Part model, mm, in its own coordinate system. Face numbers are marked on the shaded views. A direction names the side the tool comes from. Round coordinates to 2 decimals unless told otherwise and drop trailing zeros. Loops run counter-clockwise (first coordinate to the right, second up) from the corner with the lowest first, then second, coordinate; pieces in that order, holes last.
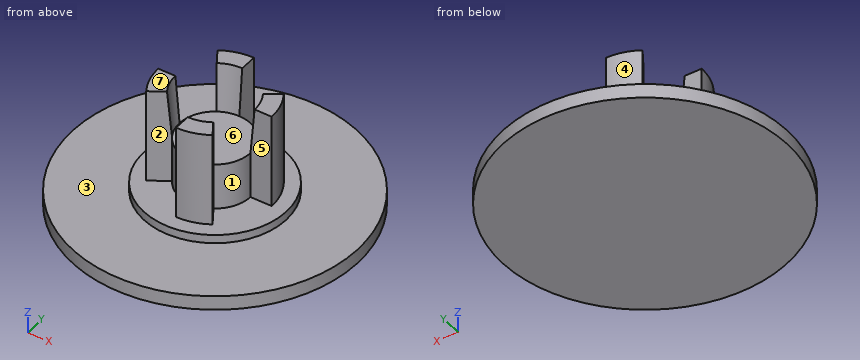
from build123d import *

# Parameters (mm, degrees)
F3_DEPTH = 6.6
F4_COUNT = 4
F5_DEPTH = 3.35
F5_TAPER = -5


with BuildPart() as f1:
    # F0 (on Front) → F1 (revolve)
    with BuildSketch(Plane.XZ):
        Polygon((0, 4.85), (0, 0), (10, 0), (10, 1), (5, 1), (5, 1.6), (2.5, 1.6), (2.5, 3.85), (2.5, 4.85), align=None)
    revolve(axis=Axis((0, 0, 2.425), (0, 0, -1)))

    # F2 (on face) → F3 (join)
    with BuildSketch(Plane.XY.offset(1.6)):
        with BuildLine():
            ThreePointArc((4, 0), (3.8409617055, 1.1166974421), (3.3764934114, 2.1445960558))
            Line((3.3764934114, 2.1445960558), (2.1103083822, 1.3403725349))
            ThreePointArc((2.1103083822, 1.3403725349), (2.4006010659, 0.6979359013), (2.5, 0))
            Line((2.5, 0), (4, 0))
        make_face()
    extrude(amount=F3_DEPTH)

    # F4: F1 ×4 about axis
    f4_axis = Axis((0, 0, 2.425), (0, 0, -1))


with BuildPart() as f1_1:
    add(f1.part)
    for i in range(1, F4_COUNT):
        add(f1.part.rotate(f4_axis, i * 360 / F4_COUNT))

    # F1_face1 (on face) → F5 (cut, through all)
    with BuildSketch(Plane.XY.offset(4.85)):
        with BuildLine():
            ThreePointArc((1.3403725349, -2.1103083822), (2.1909965013, -1.203966084), (2.5, 0))
            ThreePointArc((2.5, 0), (2.4006010659, 0.6979359013), (2.1103083822, 1.3403725349))
            ThreePointArc((2.1103083822, 1.3403725349), (1.203966084, 2.1909965013), (0, 2.5))
            ThreePointArc((0, 2.5), (-0.6979359013, 2.4006010659), (-1.3403725349, 2.1103083822))
            ThreePointArc((-1.3403725349, 2.1103083822), (-2.1909965013, 1.203966084), (-2.5, 0))
            ThreePointArc((-2.5, 0), (-2.4006010659, -0.6979359013), (-2.1103083822, -1.3403725349))
            ThreePointArc((-2.1103083822, -1.3403725349), (-1.203966084, -2.1909965013), (0, -2.5))
            ThreePointArc((0, -2.5), (0.6979359013, -2.4006010659), (1.3403725349, -2.1103083822))
        make_face()
    extrude(amount=F5_DEPTH, taper=F5_TAPER, mode=Mode.SUBTRACT)


solid = f1_1.part
1) Slice it at A-A, the plane z = 4. Give the cut face in (x, y).
Values:
outline: (-4, 0) arc R4 ccw to (-3.38, -2.14) - (-2.11, -1.34) arc R2.5 ccw to (0, -2.5) - (0, -4) arc R4 ccw to (2.14, -3.38) - (1.34, -2.11) arc R2.5 ccw to (2.5, 0) - (4, 0) arc R4 ccw to (3.38, 2.14) - (2.11, 1.34) arc R2.5 ccw to (0, 2.5) - (0, 4) arc R4 ccw to (-2.14, 3.38) - (-1.34, 2.11) arc R2.5 ccw to (-2.5, 0) - close
2) Tool access for the marked faces 5, 6 and 7: list every direction of +Z, -Z, +X, -X, +Y, -Y with a clear straight run to the whole face (end or side of a thin tool).
Values:
face 5: +Z, +X, -Y
face 6: +Z
face 7: +Z, +X, -X, +Y, -Y
3) Slice it at D-D, the plane x = -6.75. Give the cut face in (y, z), then the cut area to 3 significant figures.
Values:
outline: (-7.38, 0) - (7.38, 0) - (7.38, 1) - (-7.38, 1) - close
area: 14.8 mm2
4) Drop flat-ended pins along their axis: pin 1 Ø4 at (x, z) = (-1.5, 7) entering from -Y; pin 2 Ø1.7 at (x, z) = (-3.5, 5.5) entering from +Y; pin 3 Ø2 at (x, y) = (-3.5, 2) entering from +Z. Give the stop position or say it passes through.
Values:
pin 1: stops at y = -4
pin 2: stops at y = 0
pin 3: stops at z = 1.6
5) Slice it at C-C, the plane x = 5.25. Give the cut face in (y, z).
Values:
outline: (-8.51, 0) - (8.51, 0) - (8.51, 1) - (-8.51, 1) - close
6) Slice it at B-B, the plane z = 5.75. Give the number of separate pieces and of enclosed holes in the cut face, then the cut area to 3 significant figures.
Values:
separate pieces: 4
enclosed holes: 0
area: 10.6 mm2
7) Mould opens along Y. For the marked faces 1, 2, 3 and 4 say: released by +Y, released by -Y, zero draft, split by the parting line, or undercut.
Values:
face 1: undercut
face 2: released by -Y
face 3: zero draft
face 4: released by +Y
8) Wall check: line 1 along Z through (x, y) = (9, 2); line 2 along Z through (x, y) = (-0.5, 0); line 3 along X through (y, z) = (0.5, 6.5). Give the ranges that are in metal, low to high.
Values:
line 1: z = 0 to 1
line 2: z = 0 to 4.85
line 3: x = 2.6 to 3.97
